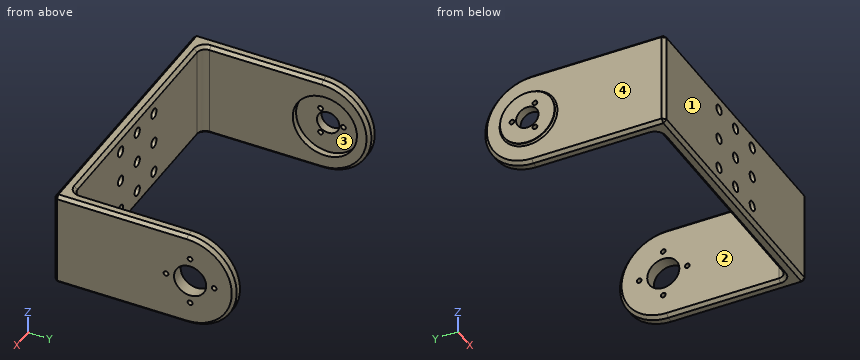
from build123d import *

# Parameters (mm, degrees)
SKETCH1_W           = 170
SKETCH1_H           = 60
BOSS_EXTRUDE1_DEPTH = 8
SKETCH2_W           = 8
SKETCH2_H           = 60
BOSS_EXTRUDE2_DEPTH = 105
SKETCH3_R           = 10
SKETCH3_R_2         = 1.5
CUT_EXTRUDE1_DEPTH  = 10
SKETCH5_R           = 17
BOSS_EXTRUDE3_DEPTH = 1.5
SKETCH6_R           = 7
CUT_EXTRUDE3_DEPTH  = 15
SKETCH7_R           = 20
CUT_EXTRUDE4_DEPTH  = 4
FILLET1_RADIUS      = 30
FILLET1_LENGTH      = 8
FILLET2_RADIUS      = 30
FILLET2_LENGTH      = 8
FILLET3_R           = 5
FILLET4_R           = 5
CHAMFER1_SIZE       = 2
SKETCH8_R           = 3.1
SKETCH8_R_2         = 3.2
CUT_EXTRUDE5_DEPTH  = 10
SKETCH10_R          = 1.5
CUT_EXTRUDE7_DEPTH  = 10
CHAMFER2_SIZE       = 1


with BuildPart() as part:
    # Sketch1 → Boss-Extrude1 (new body)
    with BuildSketch(Plane(origin=(0, 0, 0), x_dir=(1, 0, 0), z_dir=(0, 1, 0))):
        Rectangle(SKETCH1_W, SKETCH1_H)
    extrude(amount=BOSS_EXTRUDE1_DEPTH)

    # Sketch2 → Boss-Extrude2 (add)
    with BuildSketch(Plane(origin=(0, 8, 0), x_dir=(1, 0, 0), z_dir=(0, 1, 0))):
        with Locations((-81, 0)):
            Rectangle(SKETCH2_W, SKETCH2_H)
        with Locations((81, 0)):
            Rectangle(SKETCH2_W, SKETCH2_H)
    extrude(amount=BOSS_EXTRUDE2_DEPTH)

    # Sketch3 → Cut-Extrude1 (cut)
    with BuildSketch(Plane(origin=(85, 0, 0), x_dir=(0, 0, -1), z_dir=(1, 0, 0))):
        with Locations((0, 85)):
            Circle(SKETCH3_R)
        with Locations((0, 70)):
            Circle(SKETCH3_R_2)
        with Locations((0, 100)):
            Circle(SKETCH3_R_2)
        with Locations((-15, 85)):
            Circle(SKETCH3_R_2)
        with Locations((15, 85)):
            Circle(SKETCH3_R_2)
    extrude(amount=-CUT_EXTRUDE1_DEPTH, mode=Mode.SUBTRACT)

    # Sketch5 → Boss-Extrude3 (add)
    with BuildSketch(Plane.ZY.offset(85)):
        with Locations(Location((0, 85, 0), (0, 0, 180))):
            Circle(SKETCH5_R)
    extrude(amount=BOSS_EXTRUDE3_DEPTH)

    # Sketch6 → Cut-Extrude3 (cut)
    with BuildSketch(Plane.ZY.offset(86.5)):
        with Locations((0, 85)):
            Circle(SKETCH6_R)
    extrude(amount=-CUT_EXTRUDE3_DEPTH, mode=Mode.SUBTRACT)

    # Sketch7 → Cut-Extrude4 (cut)
    with BuildSketch(Plane(origin=(-77, 0, 0), x_dir=(0, 0, -1), z_dir=(1, 0, 0))):
        with Locations((0, 85)):
            Circle(SKETCH7_R)
    extrude(amount=-CUT_EXTRUDE4_DEPTH, mode=Mode.SUBTRACT)

    # Fillet1: full round fillet: the end face becomes a half cylinder, R = half its width
    fillet1_face = Plane((81, 113, 0), x_dir=(-1, 0, 0), z_dir=(0, 1, 0))  # on the end face: x along it, z out of the body
    fillet1_slab = fillet1_face.offset(-FILLET1_RADIUS / 2) * Box(FILLET1_LENGTH, 2 * FILLET1_RADIUS, FILLET1_RADIUS, mode=Mode.PRIVATE)  # the body's end, R deep
    fillet1_round = Plane((81, 83, 0), x_dir=(0, 1, 0), z_dir=(-1, 0, 0)) * Cylinder(FILLET1_RADIUS, FILLET1_LENGTH, mode=Mode.PRIVATE)  # its axis R under the face
    add(fillet1_slab - fillet1_round, mode=Mode.SUBTRACT)

    # Fillet2: full round fillet: the end face becomes a half cylinder, R = half its width
    fillet2_face = Plane((-81, 113, 0), x_dir=(1, 0, 0), z_dir=(0, 1, 0))  # on the end face: x along it, z out of the body
    fillet2_slab = fillet2_face.offset(-FILLET2_RADIUS / 2) * Box(FILLET2_LENGTH, 2 * FILLET2_RADIUS, FILLET2_RADIUS, mode=Mode.PRIVATE)  # the body's end, R deep
    fillet2_round = Plane((-81, 83, 0), x_dir=(0, 1, 0), z_dir=(1, 0, 0)) * Cylinder(FILLET2_RADIUS, FILLET2_LENGTH, mode=Mode.PRIVATE)  # its axis R under the face
    add(fillet2_slab - fillet2_round, mode=Mode.SUBTRACT)

    # Fillet3
    fillet3_edges = [part.edges().sort_by_distance(p)[0] for p in [
        (77, 8, 0),
    ]]
    fillet(fillet3_edges, radius=FILLET3_R)

    # Fillet4
    fillet4_edges = [part.edges().sort_by_distance(p)[0] for p in [
        (-77, 8, 0),
    ]]
    fillet(fillet4_edges, radius=FILLET4_R)

    # Chamfer1
    chamfer1_edges = [part.edges().sort_by_distance(p)[0] for p in [
        (75.535533906, 9.464466094, -30),
        (75.535533906, 9.464466094, 30),
        (0, 8, 30),
        (-75.535533906, 9.464466094, 30),
        (-75.535533906, 9.464466094, -30),
        (0, 0, -30),
        (85, 0, 0),
        (0, 0, 30),
        (-85, 0, 0),
        (77, 48, -30),
        (85, 41.5, -30),
        (85, 41.5, 30),
        (77, 48, 30),
        (77, 113, 0),
        (85, 113, 0),
        (-85, 41.5, -30),
        (-77, 48, -30),
        (-77, 48, 30),
        (-85, 41.5, 30),
        (-85, 113, 0),
        (-77, 113, 0),
        (0, 8, -30),
    ]]
    chamfer(chamfer1_edges, length=CHAMFER1_SIZE)

    # Sketch8 → Cut-Extrude5 (cut)
    with BuildSketch(Plane(origin=(0, 8, 0), x_dir=(1, 0, 0), z_dir=(0, 1, 0))):
        with Locations(Location((0, 0, 0), (0, 0, 270))):
            Circle(SKETCH8_R)
        with Locations(Location((0, 20, 0), (0, 0, 270))):
            Circle(SKETCH8_R)
        with Locations(Location((0, -20, 0), (0, 0, 270))):
            Circle(SKETCH8_R)
        with Locations(Location((-20, -20, 0), (0, 0, 270))):
            Circle(SKETCH8_R)
        with Locations(Location((-20, 20, 0), (0, 0, 270))):
            Circle(SKETCH8_R)
        with Locations(Location((-20, 0, 0), (0, 0, 270))):
            Circle(SKETCH8_R)
        with Locations(Location((20, -20, 0), (0, 0, 270))):
            Circle(SKETCH8_R_2)
        with Locations(Location((20, 0, 0), (0, 0, 270))):
            Circle(SKETCH8_R)
        with Locations(Location((20, 20, 0), (0, 0, 270))):
            Circle(SKETCH8_R)
    extrude(amount=-CUT_EXTRUDE5_DEPTH, mode=Mode.SUBTRACT)

    # Sketch10 → Cut-Extrude7 (cut)
    with BuildSketch(Plane(origin=(-81, 0, 0), x_dir=(0, 0, -1), z_dir=(1, 0, 0))):
        with Locations((0, 94.525)):
            Circle(SKETCH10_R)
        with Locations((8.248891971, 80.2375)):
            Circle(SKETCH10_R)
        with Locations((-8.248891971, 80.2375)):
            Circle(SKETCH10_R)
    extrude(amount=-CUT_EXTRUDE7_DEPTH, mode=Mode.SUBTRACT)

    # Chamfer2
    chamfer2_edges = [part.edges().sort_by_distance(p)[0] for p in [
        (-85, 85, 17),
    ]]
    chamfer(chamfer2_edges, length=CHAMFER2_SIZE)


solid = part.part
Verification items for the finished model (mm, model axes). Face numbers are marked on the shaded views. A direction names the side the tool comes from. Give positions to 0.01 mm unless a question says otherwise; leave off trailing zeros. Write each loop counter-clockwise with the first axis right and the second up, starting at its lowest first coordinate (ties: lowest second). Pieces come first, ordered by that corner, then holes.
(1) Material ranges on line 1 (X direction, y = 2, z = 20); line 2 (X direction, y = 4.25, z = 0); line 3 (X direction, y = 106, z = -12.5), recorded low to high.
(2) Cross-section at A-A (y = 60). Enter the section's corners in (x, z).
(3) Mould release check, pull along Z, two halves, no side actions. Record for the marked faces 3 and 4: +Z half, -Z half, draft (parallel to the pull), parting line (faces both ways), or undercut.
(4) Cross-section at B-B (x = 0). Enter the section's corners in (y, z), plus the area to 3 significant figures.
(5) Gauge pin test, flat ends, axial feed: pin 1 (3.5 mm diameter, centred on y = 85, z = 15, fed in from +X); pin 2 (17 mm diameter, centred on x = -23, z = -0.5, fed in from +Y); pin 3 (2.5 mm diameter, centred on y = 85, z = -15, fed in from +X); pin 4 (17 mm diameter, centred on y = 49, z = 3, fed in from -X). Record the tip position at first contact, or that the pin passes through.
(6) Cross-section at C-C (x = -52.5). Enter the section's corners in (y, z).
(7) Access from +Z, -Z, +X, -X, +Y, -Y to the whole of each face (thin tool, end or side, straight path). Record for the marked faces 1 and 2.
Worked out:
1. line 1: x = -85 to -23.1, -16.9 to -3.1, 3.1 to 16.8, 23.2 to 85
1. line 2: x = -85 to -23.1, -16.9 to -3.1, 3.1 to 16.9, 23.1 to 85
1. line 3: x = -85 to -77, 77 to 85
2. outline: (-85, -28) - (-83, -30) - (-79, -30) - (-77, -28) - (-77, 28) - (-79, 30) - (-83, 30) - (-85, 28) - close; (77, -28) - (79, -30) - (83, -30) - (85, -28) - (85, 28) - (83, 30) - (79, 30) - (77, 28) - close
3. face 3: undercut
3. face 4: draft
4. outline: (0, -28) - (2, -30) - (6, -30) - (8, -28) - (8, -23.1) - (0, -23.1) - close; (0, -16.9) - (8, -16.9) - (8, -3.1) - (0, -3.1) - close; (0, 3.1) - (8, 3.1) - (8, 16.9) - (0, 16.9) - close; (0, 23.1) - (8, 23.1) - (8, 28) - (6, 30) - (2, 30) - (0, 28) - close
4. area: 323 mm2
5. pin 1: stops at x = 85
5. pin 2: stops at y = 8
5. pin 3: stops at x = -81
5. pin 4: stops at x = -85
6. outline: (0, -28) - (2, -30) - (6, -30) - (8, -28) - (8, 28) - (6, 30) - (2, 30) - (0, 28) - close
7. face 1: +Z, -Z, +X, -X, -Y
7. face 2: +Z, -Z, +Y
